The model under review builds one solid part; all positions refer to its coordinate system, in mm. Face numbers are marked on the shaded views. A direction names the side the tool comes from. Coordinates: 2 decimals unless noted, no trailing zeros. Write each loop counter-clockwise with the first axis right and the second up, starting at its lowest first coordinate (ties: lowest second). Pieces come first, ordered by that corner, then holes. Notation, with made-up numbers: M 31.25,-2.75 L 46.25,-2.75 A8 cw 46.25,2.25 Z; hole C -2,56.25 d7. An arc over 180 degrees is marked long. Answer as a JSON object with one key per item and string values.
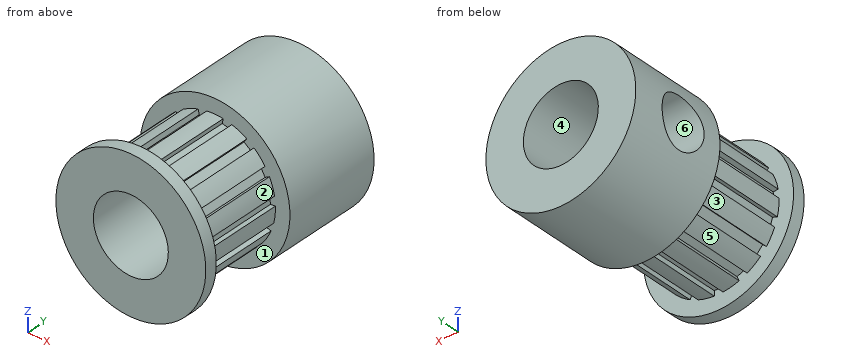
```python
from build123d import *

# Parameters (mm, degrees)
SKETCH_1_R               = 6
EXTRUDE_1_DEPTH          = 1
EXTRUDE_2_DEPTH          = 7
SKETCH_3_R               = 6
EXTRUDE_3_DEPTH          = 8
CUT_EXTRUDE_1_REACH      = 20.111
SKETCH_4_R               = 3
CUT_EXTRUDE_2_REACH      = 20.111
CUT_EXTRUDE_2_END_RADIUS = 6
SKETCH_5_R               = 2


with BuildPart() as part:
    # 草图1 → 凸台-拉伸1 (new body)
    with BuildSketch(Plane(origin=(0, 0, 0), x_dir=(1, 0, 0), z_dir=(0, 1, 0))):
        with Locations(Location((0, 0, 0), (0, 0, 270))):
            Circle(SKETCH_1_R)
    extrude(amount=EXTRUDE_1_DEPTH)

    # 草图2 → 凸台-拉伸2 (add)
    with BuildSketch(Plane(origin=(0, 1, 0), x_dir=(1, 0, 0), z_dir=(0, 1, 0))):
        with BuildLine():
            Line((-0.35, 4.427328454), (-0.35, 4.827328454))
            ThreePointArc((-0.35, 4.827328454), (-1.006292584, 4.734234388), (-1.64371046, 4.552341807))
            Line((-1.64371046, 4.552341807), (-1.481015803, 4.186923623))
            Line((-1.481015803, 4.186923623), (-2.120497623, 3.902207973))
            Line((-2.120497623, 3.902207973), (-2.28319228, 4.267626156))
            ThreePointArc((-2.28319228, 4.267626156), (-2.844880621, 3.915642253), (-3.353208449, 3.490213904))
            Line((-3.353208449, 3.490213904), (-3.055950519, 3.222561662))
            Line((-3.055950519, 3.222561662), (-3.524341943, 2.702360284))
            Line((-3.524341943, 2.702360284), (-3.821599873, 2.970012526))
            ThreePointArc((-3.821599873, 2.970012526), (-4.191562954, 2.42), (-4.482906234, 1.82459631))
            Line((-4.482906234, 1.82459631), (-4.102483628, 1.700989513))
            Line((-4.102483628, 1.700989513), (-4.318795524, 1.035249951))
            Line((-4.318795524, 1.035249951), (-4.69921813, 1.158856749))
            ThreePointArc((-4.69921813, 1.158856749), (-4.813485974, 0.505917762), (-4.837468805, -0.156510562))
            Line((-4.837468805, -0.156510562), (-4.439660047, -0.114699176))
            Line((-4.439660047, -0.114699176), (-4.366490123, -0.810864503))
            Line((-4.366490123, -0.810864503), (-4.764298881, -0.852675888))
            ThreePointArc((-4.764298881, -0.852675888), (-4.603113539, -1.495642253), (-4.355589073, -2.110555336))
            Line((-4.355589073, -2.110555336), (-4.009178912, -1.910555336))
            Line((-4.009178912, -1.910555336), (-3.659178912, -2.516773118))
            Line((-3.659178912, -2.516773118), (-4.005589073, -2.716773118))
            ThreePointArc((-4.005589073, -2.716773118), (-3.596820955, -3.238592135), (-3.120588421, -3.699665918))
            Line((-3.120588421, -3.699665918), (-2.88547432, -3.37605912))
            Line((-2.88547432, -3.37605912), (-2.319162424, -3.787508797))
            Line((-2.319162424, -3.787508797), (-2.554276525, -4.111115595))
            ThreePointArc((-2.554276525, -4.111115595), (-1.968605352, -4.421560015), (-1.346009681, -4.649070653))
            Line((-1.346009681, -4.649070653), (-1.262845005, -4.257811613))
            Line((-1.262845005, -4.257811613), (-0.578141684, -4.403349796))
            Line((-0.578141684, -4.403349796), (-0.661306361, -4.794608837))
            ThreePointArc((-0.661306361, -4.794608837), (0, -4.84), (0.661306361, -4.794608837))
            Line((0.661306361, -4.794608837), (0.578141684, -4.403349796))
            Line((0.578141684, -4.403349796), (1.262845005, -4.257811613))
            Line((1.262845005, -4.257811613), (1.346009681, -4.649070653))
            ThreePointArc((1.346009681, -4.649070653), (1.968605352, -4.421560015), (2.554276525, -4.111115595))
            Line((2.554276525, -4.111115595), (2.319162424, -3.787508797))
            Line((2.319162424, -3.787508797), (2.88547432, -3.37605912))
            Line((2.88547432, -3.37605912), (3.120588421, -3.699665918))
            ThreePointArc((3.120588421, -3.699665918), (3.596820955, -3.238592135), (4.005589073, -2.716773118))
            Line((4.005589073, -2.716773118), (3.659178912, -2.516773118))
            Line((3.659178912, -2.516773118), (4.009178912, -1.910555336))
            Line((4.009178912, -1.910555336), (4.355589073, -2.110555336))
            ThreePointArc((4.355589073, -2.110555336), (4.603113539, -1.495642253), (4.764298881, -0.852675888))
            Line((4.764298881, -0.852675888), (4.366490123, -0.810864503))
            Line((4.366490123, -0.810864503), (4.439660047, -0.114699176))
            Line((4.439660047, -0.114699176), (4.837468805, -0.156510562))
            ThreePointArc((4.837468805, -0.156510562), (4.813485974, 0.505917762), (4.69921813, 1.158856749))
            Line((4.69921813, 1.158856749), (4.318795524, 1.035249951))
            Line((4.318795524, 1.035249951), (4.102483628, 1.700989513))
            Line((4.102483628, 1.700989513), (4.482906234, 1.82459631))
            ThreePointArc((4.482906234, 1.82459631), (4.191562954, 2.42), (3.821599873, 2.970012526))
            Line((3.821599873, 2.970012526), (3.524341943, 2.702360284))
            Line((3.524341943, 2.702360284), (3.055950519, 3.222561662))
            Line((3.055950519, 3.222561662), (3.353208449, 3.490213904))
            ThreePointArc((3.353208449, 3.490213904), (2.844880621, 3.915642253), (2.28319228, 4.267626156))
            Line((2.28319228, 4.267626156), (2.120497623, 3.902207973))
            Line((2.120497623, 3.902207973), (1.481015803, 4.186923623))
            Line((1.481015803, 4.186923623), (1.64371046, 4.552341807))
            ThreePointArc((1.64371046, 4.552341807), (1.006292584, 4.734234388), (0.35, 4.827328454))
            Line((0.35, 4.827328454), (0.35, 4.427328454))
            Line((0.35, 4.427328454), (-0.35, 4.427328454))
        make_face()
    extrude(amount=EXTRUDE_2_DEPTH)

    # 草图3 → 凸台-拉伸3 (add)
    with BuildSketch(Plane(origin=(0, 8, 0), x_dir=(1, 0, 0), z_dir=(0, 1, 0))):
        with Locations(Location((0, 0, 0), (0, 0, 270))):
            Circle(SKETCH_3_R)
    extrude(amount=EXTRUDE_3_DEPTH)

    # 草图4 → 切除-拉伸1 (cut, up to next)
    with BuildSketch(Plane(origin=(0, 16, 0), x_dir=(1, 0, 0), z_dir=(0, 1, 0)), mode=Mode.PRIVATE) as cut_extrude_1_sk1:
        with Locations(Location((0, 0, 0), (0, 0, 270))):
            Circle(SKETCH_4_R)
    cut_extrude_1_tool1 = extrude(cut_extrude_1_sk1.sketch, amount=-CUT_EXTRUDE_1_REACH, mode=Mode.PRIVATE) & part.part
    add(cut_extrude_1_tool1.solids().sort_by_distance((0, 16, 0))[0], mode=Mode.SUBTRACT)

    # 切除-拉伸2: up to this cylinder (the profile starts inside it)
    cut_extrude_2_end = Plane(origin=(0, 11.5, 0), z_dir=(0, -1, 0)) * Cylinder(CUT_EXTRUDE_2_END_RADIUS, 53.222, mode=Mode.PRIVATE)
    # 草图5 → 切除-拉伸2 (cut, up to the surface)
    with BuildSketch(Plane(origin=(0, 0, 0), x_dir=(0, 0, -1), z_dir=(1, 0, 0)), mode=Mode.PRIVATE) as cut_extrude_2_sk1:
        with Locations((0, 11.5)):
            Circle(SKETCH_5_R)
    cut_extrude_2_tool1 = extrude(cut_extrude_2_sk1.sketch, amount=-CUT_EXTRUDE_2_REACH, mode=Mode.PRIVATE) & cut_extrude_2_end
    add(cut_extrude_2_tool1.solids().sort_by_distance((0, 11.5, 0))[0], mode=Mode.SUBTRACT)


solid = part.part
```
(1) Wall thickness on line 1 along Y through (x, z) = (-2, -4.75); line 2 along X through (y, z) = (1.25, -1.25); line 3 along Z through (x, y) = (2.5, 11): over which ranges is each line inside the solid? List them lowest first. Write a range as from..to.
Results list:
{"line 1": "0..1, 8..16", "line 2": "-4.25..-2.73, 2.73..4.25", "line 3": "-5.45..-1.66, 1.66..5.45"}
(2) Add section B-B on y = 14.25. Give the boundary of the cut face in (x, z).
Results list:
{"outline": "C 0,0 d12; hole C 0,0 d6"}
(3) Add section C-C on y = 11.5. Give the boundary of the cut face in (x, z), and give its area (3 significant figures).
Results list:
{"outline": "M -5.66,-2 A6 ccw long -5.66,2 L -2.24,2 A3 cw long -2.24,-2 Z", "area": "72.3 mm²"}
(4) Add section A-A on z = -0.25. Give the boundary of the cut face in (x, y).
Results list:
{"outline": "M -5.99,0 L -2.99,0 L -2.99,9.52 L -5.99,9.52 L -5.99,8 L -4.83,8 L -4.83,1 L -5.99,1 Z; M -5.99,13.48 L -2.99,13.48 L -2.99,16 L -5.99,16 Z; M 2.99,0 L 5.99,0 L 5.99,1 L 4.83,1 L 4.83,8 L 5.99,8 L 5.99,16 L 2.99,16 Z"}
(5) For pin 1 Ø3 at (x, y) = (3.5, 14) entering from +Z; pin 2 Ø4 at (x, y) = (-2, 14) entering from +Z; pin 3 Ø2 at (x, y) = (2.5, 14.5) entering from -Z; pin 4 Ø2 at (y, z) = (12.5, 4.5) entering from +X, all flat-tipped, find the tip position at first contact; note any pin that passes through.
Results list:
{"pin 1": "z = 5.66", "pin 2": "z = 6", "pin 3": "z = -5.81", "pin 4": "x = 4.87"}
(6) For the marked faces 1, 2 and 3, list the 3-axis set-ups (+Z, -Z, +X, -X, +Y, -Y) from which the entire face can be reached by the end or side of a thin tool; tool diameter is ignored.
Results list:
{"face 1": "none", "face 2": "+Z, +X", "face 3": "-Z, -X"}
(7) Draft analysis for pull direction X (two halves, no side actions). For the marked faces 4, 5 and 6, state which applies: released by +X, released by -X, zero draft, split by the parting line, or undercut.
Results list:
{"face 4": "undercut", "face 5": "released by -X", "face 6": "zero draft"}
